```python
from build123d import *

# Parameters (mm, degrees)
SKETCH1_W           = 150
SKETCH1_H           = 30
BOSS_EXTRUDE1_DEPTH = 5
SKETCH3_W           = 150
SKETCH3_H           = 5
BOSS_EXTRUDE2_DEPTH = 25
SKETCH6_R           = 5
CUT_EXTRUDE2_DEPTH  = 25
SKETCH7_R           = 2.5
CUT_EXTRUDE3_DEPTH  = 25
CHAMFER1_SIZE       = 1
FILLET2_R           = 2


with BuildPart() as part:
    # Sketch1 → Boss-Extrude1 (new body)
    with BuildSketch(Plane(origin=(0, 0, 0), x_dir=(1, 0, 0), z_dir=(0, 1, 0))):
        with Locations((22.308802864, -0.815715524)):
            Rectangle(SKETCH1_W, SKETCH1_H)
    extrude(amount=BOSS_EXTRUDE1_DEPTH)

    # Sketch3 → Boss-Extrude2 (add)
    with BuildSketch(Plane(origin=(0, 5, 0), x_dir=(1, 0, 0), z_dir=(0, 1, 0))):
        with Locations((22.308802864, 11.684284476)):
            Rectangle(SKETCH3_W, SKETCH3_H)
    extrude(amount=BOSS_EXTRUDE2_DEPTH)

    # Sketch6 → Cut-Extrude2 (cut)
    with BuildSketch(Plane(origin=(0, 5, 0), x_dir=(1, 0, 0), z_dir=(0, 1, 0))):
        with Locations(Location((82.308802864, -8.315715524, 0), (0, 0, 90))):
            Circle(SKETCH6_R)
        with Locations(Location((54.808802864, -8.315715524, 0), (0, 0, 90))):
            Circle(SKETCH6_R)
        with Locations(Location((29.808802864, -8.315715524, 0), (0, 0, 90))):
            Circle(SKETCH6_R)
        with Locations(Location((2.308802864, -8.315715524, 0), (0, 0, 90))):
            Circle(SKETCH6_R)
        with Locations(Location((-37.691197136, -8.315715524, 0), (0, 0, 90))):
            Circle(SKETCH6_R)
    extrude(amount=-CUT_EXTRUDE2_DEPTH, mode=Mode.SUBTRACT)

    # Sketch7 → Cut-Extrude3 (cut)
    with BuildSketch(Plane.XY.offset(-9.184284476)):
        with Locations((82.308802864, 17.478664245)):
            Circle(SKETCH7_R)
        with Locations((-37.691197136, 17.478664245)):
            Circle(SKETCH7_R)
        with Locations((22.308802864, 17.478664245)):
            Circle(SKETCH7_R)
    extrude(amount=-CUT_EXTRUDE3_DEPTH, mode=Mode.SUBTRACT)

    # Chamfer1
    chamfer1_edges = [part.edges().sort_by_distance(p)[0] for p in [
        (79.808802864, 17.478664245, -9.184284476),
        (-40.191197136, 17.478664245, -9.184284476),
        (19.808802864, 17.478664245, -9.184284476),
    ]]
    chamfer(chamfer1_edges, length=CHAMFER1_SIZE)

    # Fillet2
    fillet2_edges = [part.edges().sort_by_distance(p)[0] for p in [
        (22.308802864, 5, 15.815715524),
        (22.308802864, 0, 15.815715524),
        (22.308802864, 5, -9.184284476),
        (-52.691197136, 30, -11.684284476),
        (97.308802864, 30, -11.684284476),
    ]]
    fillet(fillet2_edges, radius=FILLET2_R)


solid = part.part
```
Input: part model. Units: mm. Frame: model coordinates. A direction names the side the tool comes from. Round coordinates to 2 decimals unless told otherwise and drop trailing zeros. Write each loop counter-clockwise with the first axis right and the second up, starting at its lowest first coordinate (ties: lowest second). Pieces come first, ordered by that corner, then holes. Notation, with made-up numbers: M -29.5,-37 L -22.5,-37 A9 cw -22.5,-26 Z; hole C 82,32 d3. An arc over 180 degrees is marked long. Write each question's results on one line, items separated by ' | '.
Q1. Line query: line 1 along X through (y, z) = (18.5, -11.25); line 2 along Z through (x, y) = (18, 21.75); line 3 along Y through (x, z) = (67, 5.25). Output: solid intervals per line, ascending.
Results:
line 1: x = -52.69 to -39.97, -35.41 to 20.03, 24.59 to 80.03, 84.59 to 97.31 | line 2: z = -14.18 to -9.18 | line 3: y = 0 to 5
Q2. Access query for faces 1 (the face through (21, 5, 3)), 2 (the face through (21, 15, -14.184)). Directions: +Z, -Z, +X, -X, +Y, -Y. A direction counts if a zero-diameter tool reaches every point of the face in a straight line with its end or side. Return the directions, or none.
Results:
face 1: +Z, +X, -X, +Y | face 2: -Z, +X, -X, +Y, -Y
Q3. Draft query along Y for faces 3 (the face through (78.93, 2.54, 12)), 4 (the face through (21, 30, -12)), 5 (the face through (84.693, 18.23, -12.156)). Return one class per face: released by +Y, released by -Y, zero draft, split by the parting line, or undercut.
Results:
face 3: zero draft | face 4: released by +Y | face 5: undercut
Q4. Section query A-A (x = 28). Return loops of the section in (y, z), and give its area (3 significant figures).
Results:
outline: M 0,-14.18 L 30,-14.18 L 30,-9.18 L 7,-9.18 A2 cw 5,-7.18 L 5,3.65 L 0,3.65 Z; M 0,12.98 L 5,12.98 L 5,13.82 A2 ccw 3,15.82 L 2,15.82 A2 ccw 0,13.82 Z | area: 228 mm^2
Q5. Section query D-D (x = 47). Return loops of the section in (y, z), and give its area (3 significant figures).
Results:
outline: M 0,-14.18 L 30,-14.18 L 30,-9.18 L 7,-9.18 A2 cw 5,-7.18 L 5,13.82 A2 ccw 3,15.82 L 2,15.82 A2 ccw 0,13.82 Z | area: 274 mm^2
Q6. Section query B-B (z = 11.25). Return loops of the section in (x, y).
Results:
outline: M -52.69,0 L -41.74,0 L -41.74,5 L -52.69,5 Z; M -33.64,0 L -1.74,0 L -1.74,5 L -33.64,5 Z; M 6.36,0 L 25.76,0 L 25.76,5 L 6.36,5 Z; M 33.86,0 L 50.76,0 L 50.76,5 L 33.86,5 Z; M 58.86,0 L 78.26,0 L 78.26,5 L 58.86,5 Z; M 86.36,0 L 97.31,0 L 97.31,5 L 86.36,5 Z
Q7. Pin query (flat end, axial travel): P1, Ø16, axis at x = -37.69, z = 8.32, coming from the +Y side; P2, Ø1, axis at x = -11.5, z = 4, coming from the -Y side; P3, Ø6, axis at x = -37.69, y = 17.48, coming from the +Z side. Return the tip coordinate at first contact, or that it passes through.
Results:
P1: stops at y = 5 | P2: stops at y = 0 | P3: stops at z = -9.68
Q8. Section query C-C (y = 10.25). Return loops of the section in (x, z), and give its area (3 significant figures).
Results:
outline: M -52.69,-14.18 L 97.31,-14.18 L 97.31,-9.18 L -52.69,-9.18 Z | area: 750 mm^2
